Geometry: final body of the model. Coordinates: model frame, mm. A direction names the side the tool comes from. Give positions to 0.01 mm unless a question says otherwise; leave off trailing zeros. Write each loop counter-clockwise with the first axis right and the second up, starting at its lowest first coordinate (ties: lowest second). Pieces come first, ordered by that corner, then holes. Notation, with made-up numbers: M -31,-15 L -26,-15 A14 ccw -26,-2 Z; hole C 3,67.5 d8. An arc over 180 degrees is marked long. Use a Markdown table: item, result. Add a question column.
1) Pin query (flat end, axial travel): pin 1 (3.5 mm diameter, centred on y = 13, z = -0.73, fed in from -X); pin 2 (1.8 mm diameter, centred on y = 13, z = -0.73, fed in from +X); pin 3 (4 mm diameter, centred on x = 2.7, z = 4.22, fed in from +Y). Return the tip coordinate at first contact, or that it passes through.
2) Set-up query: faces 1 (the flat face through (7, 2, 5)), 2 (the flat face through (6, 1, -13.231)). Return all of +Z, -Z, +X, -X, +Y, -Y with unobstructed straight access to the full face (end or side cutting, diameter ignored); none if empty.
3) Section D-D on x = -10. Return the cut outline in (y, z).
4) Section C-C on z = -3. Return the cut outline in (x, y), then the cut area to 3 significant figures.
5) Line query: line 1 (X direction, y = 15.5, z = 10.5); line 2 (Y direction, x = 29.5, z = -9.5). Output: solid intervals per line, ascending.
6) Draft query along Y for faces 3 (the flat face through (35.654, 17, -4)), 4 (the flat face through (7, 0, -6)), 5 (the cylindrical face through (-19.36, 21.01, 5.16)). Return one class per face: +Y half, -Y half, draft (parallel to the pull), parting line (faces both ways), or undercut.
7) Section A-A on y = 10. Return the cut outline in (x, z).
8) Section B-B on y = 27. Return the cut outline in (x, z).
```python
from build123d import *

# Parameters (mm, degrees)
SKETCH_1_W          = 56
SKETCH_1_H          = 25
EXTRUDE_1_DEPTH     = 2
SKETCH_2_R          = 3
SKETCH_2_R_2        = 1.5
CUT_EXTRUDE_1_DEPTH = 39.082744359
EXTRUDE_2_DEPTH     = 2
CUT_EXTRUDE_2_REACH = 68.086
SKETCH_4_R          = 4
SKETCH_4_R_2        = 1.5
FILLET_1_R          = 1


with BuildPart() as part:
    # Sketch 1 → Extrude 1 (new body)
    with BuildSketch(Plane(origin=(0, 0, 0), x_dir=(1, 0, 0), z_dir=(0, 1, 0))):
        with Locations((7.654255319, 0.731382979)):
            Rectangle(SKETCH_1_W, SKETCH_1_H)
    extrude(amount=EXTRUDE_1_DEPTH)

    # Sketch 2 → Cut-Extrude 1 (cut, through all)
    with BuildSketch(Plane(origin=(0, 2, 0), x_dir=(1, 0, 0), z_dir=(0, 1, 0))):
        with Locations(Location((7.654255319, 0.731382979, 0), (0, 0, 270))):
            Circle(SKETCH_2_R)
        with Locations(Location((12.604002787, 5.681130447, 0), (0, 0, 270))):
            Circle(SKETCH_2_R_2)
        with Locations(Location((2.704507851, 5.681130447, 0), (0, 0, 270))):
            Circle(SKETCH_2_R_2)
        with Locations(Location((12.604002787, -4.21836449, 0), (0, 0, 270))):
            Circle(SKETCH_2_R_2)
        with Locations(Location((2.704507851, -4.21836449, 0), (0, 0, 270))):
            Circle(SKETCH_2_R_2)
    extrude(amount=-CUT_EXTRUDE_1_DEPTH, mode=Mode.SUBTRACT)

    # Sketch 3 → Extrude 2 (add)
    with BuildSketch(Plane.ZY.offset(20.345744681)):
        with BuildLine():
            Line((-13.231382979, 20), (-13.231382979, 2))
            Line((-13.231382979, 2), (11.768617021, 2))
            Line((11.768617021, 2), (11.768617021, 20))
            ThreePointArc((11.768617021, 20), (-0.731382979, 32.5), (-13.231382979, 20))
        make_face()
    extrude_2 = extrude(amount=-EXTRUDE_2_DEPTH)

    # Sketch 4 → Cut-Extrude 2 (cut, up to next)
    with BuildSketch(Plane.ZY.offset(20.345744681), mode=Mode.PRIVATE) as cut_extrude_2_sk1:
        with Locations((-0.731382979, 20)):
            Circle(SKETCH_4_R)
    cut_extrude_2_tool1 = extrude(cut_extrude_2_sk1.sketch, amount=-CUT_EXTRUDE_2_REACH, mode=Mode.PRIVATE) & part.part
    # Sketch 4 → Cut-Extrude 2 (cut, up to next)
    with BuildSketch(Plane.ZY.offset(20.345744681), mode=Mode.PRIVATE) as cut_extrude_2_sk2:
        with Locations((-0.731382979, 27)):
            Circle(SKETCH_4_R_2)
    cut_extrude_2_tool2 = extrude(cut_extrude_2_sk2.sketch, amount=-CUT_EXTRUDE_2_REACH, mode=Mode.PRIVATE) & part.part
    # Sketch 4 → Cut-Extrude 2 (cut, up to next)
    with BuildSketch(Plane.ZY.offset(20.345744681), mode=Mode.PRIVATE) as cut_extrude_2_sk3:
        with Locations((6.268617021, 20)):
            Circle(SKETCH_4_R_2)
    cut_extrude_2_tool3 = extrude(cut_extrude_2_sk3.sketch, amount=-CUT_EXTRUDE_2_REACH, mode=Mode.PRIVATE) & part.part
    # Sketch 4 → Cut-Extrude 2 (cut, up to next)
    with BuildSketch(Plane.ZY.offset(20.345744681), mode=Mode.PRIVATE) as cut_extrude_2_sk4:
        with Locations((-0.731382979, 13)):
            Circle(SKETCH_4_R_2)
    cut_extrude_2_tool4 = extrude(cut_extrude_2_sk4.sketch, amount=-CUT_EXTRUDE_2_REACH, mode=Mode.PRIVATE) & part.part
    # Sketch 4 → Cut-Extrude 2 (cut, up to next)
    with BuildSketch(Plane.ZY.offset(20.345744681), mode=Mode.PRIVATE) as cut_extrude_2_sk5:
        with Locations((-7.731382979, 20)):
            Circle(SKETCH_4_R_2)
    cut_extrude_2_tool5 = extrude(cut_extrude_2_sk5.sketch, amount=-CUT_EXTRUDE_2_REACH, mode=Mode.PRIVATE) & part.part
    cut_extrude_2_1 = cut_extrude_2_tool1.solids().sort_by_distance((-20.345745, 20, -0.731383))[0]
    add(cut_extrude_2_1, mode=Mode.SUBTRACT)
    cut_extrude_2_2 = cut_extrude_2_tool2.solids().sort_by_distance((-20.345745, 27, -0.731383))[0]
    add(cut_extrude_2_2, mode=Mode.SUBTRACT)
    cut_extrude_2_3 = cut_extrude_2_tool3.solids().sort_by_distance((-20.345745, 20, 6.268617))[0]
    add(cut_extrude_2_3, mode=Mode.SUBTRACT)
    cut_extrude_2_4 = cut_extrude_2_tool4.solids().sort_by_distance((-20.345745, 13, -0.731383))[0]
    add(cut_extrude_2_4, mode=Mode.SUBTRACT)
    cut_extrude_2_5 = cut_extrude_2_tool5.solids().sort_by_distance((-20.345745, 20, -7.731383))[0]
    add(cut_extrude_2_5, mode=Mode.SUBTRACT)
    cut_extrude_2 = cut_extrude_2_1 + cut_extrude_2_2 + cut_extrude_2_3 + cut_extrude_2_4 + cut_extrude_2_5  # Cut-Extrude 2 as one shape, for the pattern or mirror that repeats it

    # Mirror 1: Extrude 2, Cut-Extrude 2 across plane
    add(extrude_2.mirror(Plane.ZY.offset(-7.654255319)))
    add(cut_extrude_2.mirror(Plane.ZY.offset(-7.654255319)), mode=Mode.SUBTRACT)

    # Fillet 1
    fillet_1_edges = [part.edges().sort_by_distance(p)[0] for p in [
        (35.654255319, 0, -0.731382979),
        (-20.345744681, 0, -0.731382979),
    ]]
    fillet(fillet_1_edges, radius=FILLET_1_R)


solid = part.part
```
Found:
| question | item | result |
|---|---|---|
| 1 | pin 1 | x = -20.35 |
| 1 | pin 2 | through |
| 1 | pin 3 | y = 2 |
| 2 | face 1 | +Z, -Z, +Y |
| 2 | face 2 | -Z, +X, -X, +Y, -Y |
| 3 | outline | M 0,-13.23 L 2,-13.23 L 2,11.77 L 0,11.77 Z |
| 4 | outline | M -20.35,1 A1 ccw -19.35,0 L 5.69,0 L 5.69,2 L -18.35,2 L -18.35,16.71 L -20.35,16.71 Z; M -20.35,23.29 L -18.35,23.29 L -18.35,32.29 L -20.35,32.29 Z; M 9.62,0 L 34.65,0 A1 ccw 35.65,1 L 35.65,16.71 L 33.65,16.71 L 33.65,2 L 9.62,2 Z; M 33.65,23.29 L 35.65,23.29 L 35.65,32.29 L 33.65,32.29 Z |
| 4 | area | 199 mm² |
| 5 | line 1 | -20.35 to -18.35, 33.65 to 35.65 |
| 5 | line 2 | 0 to 2 |
| 6 | face 3 | draft |
| 6 | face 4 | -Y half |
| 6 | face 5 | undercut |
| 7 | outline | M -20.35,-13.23 L -18.35,-13.23 L -18.35,11.77 L -20.35,11.77 Z; M 33.65,-13.23 L 35.65,-13.23 L 35.65,11.77 L 33.65,11.77 Z |
| 8 | outline | M -20.35,-11.09 L -18.35,-11.09 L -18.35,-2.23 L -20.35,-2.23 Z; M -20.35,0.77 L -18.35,0.77 L -18.35,9.62 L -20.35,9.62 Z; M 33.65,-11.09 L 35.65,-11.09 L 35.65,-2.23 L 33.65,-2.23 Z; M 33.65,0.77 L 35.65,0.77 L 35.65,9.62 L 33.65,9.62 Z |
